```python
from build123d import *

# Parameters (mm, degrees)
SKETCH1_W                = 41
SKETCH1_H                = 29
BOSS_EXTRUDE1_DEPTH      = 3
SKETCH11_R               = 3
BOSS_EXTRUDE2_DEPTH      = 1.5
F_4_0_4_DIAMETER_HOLE1_D = 4


with BuildPart() as part:
    # Sketch1 → Boss-Extrude1 (new body)
    with BuildSketch(Plane.XY):
        Rectangle(SKETCH1_W, SKETCH1_H)
    extrude(amount=BOSS_EXTRUDE1_DEPTH)


with BuildPart() as part_1:
    # Body-Move/Copy1: moved
    add(part.part.moved(Location((0.5, 0.5, 0))))

    # Sketch11 → Boss-Extrude2 (add)
    with BuildSketch(Plane.XY.offset(3)):
        with Locations((-9.387244392, 0.5)):
            Circle(SKETCH11_R)
        with Locations((10.452938647, 0.5)):
            Circle(SKETCH11_R)
    extrude(amount=BOSS_EXTRUDE2_DEPTH)

    # Ø4.0 (4) Diameter Hole1 (through all)
    with Locations(Plane.XY.offset(4.5)):
        with Locations((-9.387244392, 0.5), (10.452938647, 0.5)):
            Hole(F_4_0_4_DIAMETER_HOLE1_D / 2)


with BuildPart() as part_2:
    # Body-Move/Copy8: moved
    add(part_1.part.moved(Location((27.795693281, 0, 0))))


solid = part_2.part
```
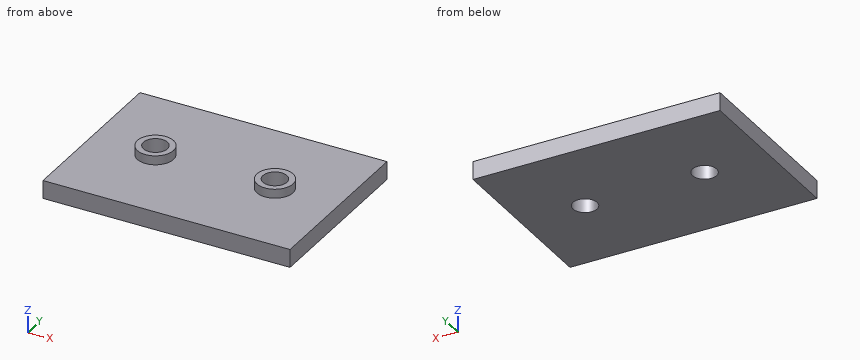
For this review, take the finished solid that the model builds, in its own axes (mm). Coordinates: 2 decimals unless noted, no trailing zeros. Write each loop counter-clockwise with the first axis right and the second up, starting at its lowest first coordinate (ties: lowest second). Pieces come first, ordered by that corner, then holes.
(1) Add section C-C on x = 29. Give the boundary of the cut face in (y, z), then the cut area to 3 significant figures.
(2) Wall thickness on probe 1 along Z at (x, y) = (14, 10); probe 2 along Y at (x, z) = (37, 0.2); probe 3 along Y at (x, z) = (17, 2.25): over which ranges is each line inside the solid? List them lowest first.
(3) Add section D-D on y = -8. Give the boundary of the cut face in (x, z), then the cut area to 3 significant figures.
(4) For pin 1 Ø3 at (x, y) = (31, 7.5) entering from +Z, flat-tipped, find the tip position at first contact; note if it passes through.
(5) Add section A-A on y = 0.5. Give the boundary of the cut face in (x, z), then the cut area to 3 significant figures.
(6) Add section B-B on z = 3.5. Give the boundary of the cut face in (x, y).
Answer sheet:
1. outline: (-14, 0) - (15, 0) - (15, 3) - (-14, 3) - close
1. area: 87.0 mm2
2. probe 1: z = 0 to 3
2. probe 2: y = -14 to -1.06, 2.06 to 15
2. probe 3: y = -14 to -0.92, 1.92 to 15
3. outline: (7.8, 0) - (48.8, 0) - (48.8, 3) - (7.8, 3) - close
3. area: 123 mm2
4. pin 1: stops at z = 3
5. outline: (7.8, 0) - (16.41, 0) - (16.41, 4.5) - (15.41, 4.5) - (15.41, 3) - (7.8, 3) - close; (20.41, 0) - (36.25, 0) - (36.25, 4.5) - (35.25, 4.5) - (35.25, 3) - (21.41, 3) - (21.41, 4.5) - (20.41, 4.5) - close; (40.25, 0) - (48.8, 0) - (48.8, 3) - (41.25, 3) - (41.25, 4.5) - (40.25, 4.5) - close
5. area: 105 mm2
6. outline: circle Ø6 at (18.41, 0.5); circle Ø6 at (38.25, 0.5); hole circle Ø4 at (18.41, 0.5); hole circle Ø4 at (38.25, 0.5)
